Check sheet for the modelled part. Datum: model origin and axes. Units: mm. A direction names the side the tool comes from. Give positions to 0.01 mm unless a question says otherwise; leave off trailing zeros. Loops run counter-clockwise (first coordinate to the right, second up) from the corner with the lowest first, then second, coordinate; pieces in that order, holes last. Notation, with made-up numbers: (27.5, -7) - (48.5, -7) arc R17 cw to (48.5, 1) - close; hole circle Ø7 at (-28, -27). An arc over 180 degrees is marked (long way). Answer in a Markdown table with one row per item. Add a question column.
(1) Set-up check for faces 5 (the face through (15.5, 0, -1)), 6 (the face through (-2.623, 9.278, -3.986)), 7 (the face through (0, 0, 0)), 8 (the face through (0, 32, 22)): record each of +Z, -Z, +X, -X, +Y, -Y from which the full face is reachable in a straight line by a thin tool's end or side.
(2) Go/stop test with flat-tipped pins: P1, Ø0.9, axis at y = -15, z = -1, coming from the +X side; P2, Ø8, axis at x = 0, y = 26, coming from the +Z side; P3, Ø5, axis at x = -3, y = 12.5, coming from the -Z side. Record where each tip stops, or that it passes through.
(3) Sectioned sample at B-B on x = 8.5. Enter the section's corners in (y, z), then the cut area to 4 significant figures.
(4) Sectioned sample at C-C on y = 12.5. Enter the section's corners in (x, z), then the cut area to 3 significant figures.
(5) Thickness scan on L1, parallel to X at y = 0, z = -2; L2, parallel to X at y = 12.5, z = -3.9; L3, parallel to Z at x = -5, y = 23.5. Record the ranges inside material, lowest first.
(6) Draft check along X on faces 1 (the face through (18.25, 31.98, -22.19)), 2 (the face through (-0.8, 12.5, -5)), 3 (the face through (-20.87, 31.98, 19.5)), 4 (the face through (-15.5, 0, -1)). Enter one of: released by +X, released by -X, zero draft, split by the parting line, or undercut.
(7) Sectioned sample at D-D on x = -2. Enter the section's corners in (y, z), then the cut area to 3 significant figures.
(8) Sectioned sample at A-A on y = 0. Enter the section's corners in (x, z), then the cut area to 3 significant figures.
from build123d import *

# Parameters (mm, degrees)
SKETCH_R        = 1.25
PAD_DEPTH       = 3
SKETCH002_W     = 44
SKETCH002_H     = 48
PAD001_DEPTH    = 3
SKETCH006_R     = 1.6
POCKET001_DEPTH = 3
SKETCH007_R     = 3.25
PAD004_DEPTH    = 2
SKETCH008_R     = 1.25
POCKET002_DEPTH = 5


with BuildPart() as part:
    # Sketch (on Face1 of Binder) → Pad (new body)
    with BuildSketch(Plane(origin=(0, 0, 0), x_dir=(1, 0, 0), z_dir=(0, 0, -1))):
        Polygon((-15.5, 28.5), (-15.5, -28.5), (-15.5, -30.5), (15.5, -30.5), (15.5, -28.5), (15.5, 28.5), (15.5, 30.5), (-15.5, 30.5), align=None)
        with Locations((-8.5, 0)):
            Circle(SKETCH_R, mode=Mode.SUBTRACT)
        with Locations((8.5, 0)):
            Circle(SKETCH_R, mode=Mode.SUBTRACT)
    extrude(amount=PAD_DEPTH)

    # Sketch002 (on Face1 of Pad) → Pad001 (join)
    with BuildSketch(Plane(origin=(0, 30.5, 0), x_dir=(-1, 0, 0), z_dir=(0, 1, 0))):
        with Locations((0, -2)):
            Rectangle(SKETCH002_W, SKETCH002_H)
    extrude(amount=PAD001_DEPTH)

    # Sketch006 (on Face3 of Pad001) → Pocket001 (cut)
    with BuildSketch(Plane.XZ.offset(-30.5)):
        with Locations((-19.271234, 19.432414)):
            Circle(SKETCH006_R)
        with Locations((19.462404, 19.260412)):
            Circle(SKETCH006_R)
        with Locations((19.428404, -23.271234)):
            Circle(SKETCH006_R)
        with Locations((-19.271234, -23.428404)):
            Circle(SKETCH006_R)
    extrude(amount=-POCKET001_DEPTH, mode=Mode.SUBTRACT)

    # Sketch007 (on Face8 of Pocket001) → Pad004 (join)
    with BuildSketch(Plane(origin=(0, 0, -3), x_dir=(1, 0, 0), z_dir=(0, 0, -1))):
        with Locations((-2.2, -12.5)):
            Circle(SKETCH007_R)
    extrude(amount=PAD004_DEPTH)

    # Sketch008 (on Face19 of Pad004) → Pocket002 (cut)
    with BuildSketch(Plane(origin=(0, 0, -5), x_dir=(1, 0, 0), z_dir=(0, 0, -1))):
        with Locations((-2.2, -12.5)):
            Circle(SKETCH008_R)
    extrude(amount=-POCKET002_DEPTH, mode=Mode.SUBTRACT)


solid = part.part
Reply:
| question | item | result |
|---|---|---|
| 1 | face 5 | +Z, -Z, +X, -Y |
| 1 | face 6 | -Z |
| 1 | face 7 | +Z, +X, -X, -Y |
| 1 | face 8 | +Z, +X, -X, +Y, -Y |
| 2 | P1 | x = 15.5 |
| 2 | P2 | z = 0 |
| 2 | P3 | z = -5 |
| 3 | outline | (-30.5, -3) - (-1.25, -3) - (-1.25, 0) - (-30.5, 0) - close; (1.25, -3) - (30.5, -3) - (30.5, -26) - (33.5, -26) - (33.5, 22) - (30.5, 22) - (30.5, 0) - (1.25, 0) - close |
| 3 | area | 319.5 mm^2 |
| 4 | outline | (-15.5, -3) - (-5.45, -3) - (-5.45, -5) - (-3.45, -5) - (-3.45, 0) - (-15.5, 0) - close; (-0.95, -5) - (1.05, -5) - (1.05, -3) - (15.5, -3) - (15.5, 0) - (-0.95, 0) - close |
| 4 | area | 93.5 mm^2 |
| 5 | L1 | -15.5 to -9.75, -7.25 to 7.25, 9.75 to 15.5 |
| 5 | L2 | -5.45 to -3.45, -0.95 to 1.05 |
| 5 | L3 | -3 to 0 |
| 6 | face 1 | undercut |
| 6 | face 2 | zero draft |
| 6 | face 3 | undercut |
| 6 | face 4 | released by -X |
| 7 | outline | (-30.5, -3) - (9.26, -3) - (9.26, -5) - (11.27, -5) - (11.27, 0) - (-30.5, 0) - close; (13.73, -5) - (15.74, -5) - (15.74, -3) - (30.5, -3) - (30.5, -26) - (33.5, -26) - (33.5, 22) - (30.5, 22) - (30.5, 0) - (13.73, 0) - close |
| 7 | area | 328 mm^2 |
| 8 | outline | (-15.5, -3) - (-9.75, -3) - (-9.75, 0) - (-15.5, 0) - close; (-7.25, -3) - (7.25, -3) - (7.25, 0) - (-7.25, 0) - close; (9.75, -3) - (15.5, -3) - (15.5, 0) - (9.75, 0) - close |
| 8 | area | 78.0 mm^2 |
